Autodesk Fusion 360 part; units mm, degrees
sketch "Sketch1" plane through (0, 0, 0) normal (0, 1, 0) x (1, 0, 0)
  circle A0 centre (0, 0) radius 4.075
  line L0 (26.5, -2.5) -> (17.4, -2.5)
  line L1 (17.4, -2.5) -> (17.4, 2.5)
  line L2 (17.4, 2.5) -> (26.5, 2.5)
  line L3 (26.5, 2.5) -> (26.5, -2.5)
  line L4 (26.5, -2.5) -> (17.4, 2.5) construction
  line L5 (17.4, -2.5) -> (26.5, 2.5) construction
  circle A1 centre (13, 0) radius 2
  circle A2 centre (31, 0) radius 2
  line L6 (-10, 10) -> (41, 10)
  line L7 (41, 10) -> (41, -10)
  line L8 (41, -10) -> (-10, -10)
  line L9 (-10, -10) -> (-10, 10)
  line L10 (-10, 10) -> (-12, 10)
  line L11 (-12, 10) -> (-12, -10)
  line L12 (-12, -10) -> (-10, -10)
  line L13 (-10, -10) -> (-10, 10)
  line L14 (41, 10) -> (43, 10)
  line L15 (43, 10) -> (43, -10)
  line L16 (43, -10) -> (41, -10)
  line L17 (41, -10) -> (41, 10)
  point P0 (21.95, 0)
  dimension "d1" = 8.15
  dimension "d2" = 9.1
  dimension "d3" = 5
  dimension "d4" = 4
  dimension "d5" = 4
  dimension "d6" = 18
  dimension "d7" = 9.05
  dimension "d9" = 13
  dimension "d10" = 10
  dimension "d11" = 10
  dimension "d12" = 10
  dimension "d13" = 10
  dimension "d16" = 51
extrude "Extrude2" add sketch "Sketch1" along normal blind 2 contours L6 L7 L8 L9 L13 L17 makes body 1
extrude "Extrude1" add sketch "Sketch1" along normal blind 2 separate body contours L6 L7 L8 L9 L13 L17 makes body 2
extrude "Extrude3" add sketch "Sketch1" along normal blind 55 contours L9 L10 L11 L12 L13 | L7 L14 L15 L16 L17 bodies 1 2
sketch "Sketch2" plane through (-10, 0, 0) normal (1, 0, 0) x (0, 0, -1)
  line L0 (-10, 2) -> (10, 2)
  line L1 (10, 2) -> (10, 55)
  line L2 (10, 55) -> (-10, 55)
  line L3 (-10, 55) -> (-10, 2)
  line L4 (-10, 55) -> (10, 55)
  line L5 (10, 55) -> (10, 53)
  line L6 (10, 53) -> (-10, 53)
  line L7 (-10, 53) -> (-10, 55)
  dimension "d21" = 2
extrude "Extrude4" add sketch "Sketch2" along normal up to surface (51 mm away) contours L1 L2 L3 L4 L5 L6 L7 bodies 1
sketch "Sketch3" plane through (0, 0, 10) normal (0, 0, 1) x (1, 0, 0)
  line L0 (41, 53) -> (41, 2)
  line L1 (41, 2) -> (-10, 2)
  line L2 (-10, 2) -> (-10, 53)
  line L3 (-10, 53) -> (41, 53)
  line L4 (43, 55) -> (-12, 55)
  line L5 (-12, 55) -> (-12, 0)
  line L6 (-12, 0) -> (43, 0)
  line L7 (43, 0) -> (43, 55)
extrude "Extrude5" add sketch "Sketch3" along normal blind 2 contours L0 L1 L2 L3 | L4 L5 L6 L7 bodies 1
sketch "Sketch4" plane through (0, 0, -10) normal (0, 0, -1) x (-1, 0, 0)
  line L0 (12, 55) -> (-43, 55)
  line L1 (-43, 55) -> (-43, 0)
  line L2 (-43, 0) -> (12, 0)
  line L3 (12, 0) -> (12, 55)
  line L4 (-41, 53) -> (10, 53)
  line L5 (10, 53) -> (10, 2)
  line L6 (10, 2) -> (-41, 2)
  line L7 (-41, 2) -> (-41, 53)
extrude "Extrude6" add sketch "Sketch4" along normal blind 14 bodies 1
sketch "Sketch5" plane through (43, 0, 0) normal (1, 0, 0) x (0, 0, -1)
  line L0 (-12, 0) -> (24, 0)
  line L1 (24, 0) -> (24, 55)
  line L2 (24, 55) -> (-12, 55)
  line L3 (-12, 55) -> (-12, 0)
  line L4 (24, 55) -> (22, 55)
  line L5 (22, 55) -> (22, 0)
  line L6 (22, 0) -> (24, 0)
  line L7 (24, 0) -> (24, 55)
extrude "Extrude7" add sketch "Sketch5" along normal blind 5 contours L0 L1 L2 L4 L5 L6 L7 bodies 1
sketch "Sketch6" plane through (-12, 0, 0) normal (-1, 0, 0) x (0, 0, 1)
  line L0 (-24, 0) -> (12, 0)
  line L1 (12, 0) -> (12, 55)
  line L2 (12, 55) -> (-24, 55)
  line L3 (-24, 55) -> (-24, 0)
  line L4 (-24, 55) -> (-22, 55)
  line L5 (-22, 55) -> (-22, 0)
  line L6 (-22, 0) -> (-24, 0)
  line L7 (-24, 0) -> (-24, 55)
  point P0 (-22, 0)
extrude "Extrude8" add sketch "Sketch6" along normal blind 5 contours L0 L2 L3 L4 L5 L6 L7 bodies 1
sketch "Sketch7" plane through (0, 55, 0) normal (0, 1, 0) x (-1, 0, 0)
  line L0 (-48, -24) -> (17, -24)
  line L1 (17, -24) -> (17, -22)
  line L2 (17, -22) -> (12, -22)
  line L3 (12, -22) -> (12, 12)
  line L4 (12, 12) -> (-43, 12)
  line L5 (-43, 12) -> (-43, -22)
  line L6 (-43, -22) -> (-48, -22)
  line L7 (-48, -22) -> (-48, -24)
  line L8 (17, -22) -> (-48, -22)
  line L9 (-48, -22) -> (-48, -24)
  line L10 (-48, -24) -> (17, -24)
  line L11 (17, -24) -> (17, -22)
extrude "Extrude9" add sketch "Sketch7" along normal blind 5 contours L0 L1 L2 L6 L7 L8 L9 L10 L11 bodies 1
sketch "Sketch8" plane through (0, 0, 0) normal (0, -1, 0) x (1, 0, 0)
  circle A0 centre (0, 0) radius 4.075
  circle A1 centre (31, 0) radius 2
  line L0 (26.5, -2.5) -> (17.4, -2.5)
  line L1 (17.4, -2.5) -> (17.4, 2.5)
  line L2 (17.4, 2.5) -> (26.5, 2.5)
  line L3 (26.5, 2.5) -> (26.5, -2.5)
  circle A2 centre (13, 0) radius 2
  line L4 (-12, 12) -> (-12, -22)
  line L5 (-12, -22) -> (-17, -22)
  line L6 (-17, -22) -> (-17, -24)
  line L7 (-17, -24) -> (48, -24)
  line L8 (48, -24) -> (48, -22)
  line L9 (48, -22) -> (43, -22)
  line L10 (43, -22) -> (43, 12)
  line L11 (43, 12) -> (-12, 12)
  line L12 (-17, -24) -> (48, -24)
  line L13 (48, -24) -> (48, -22)
  line L14 (48, -22) -> (-17, -22)
  line L15 (-17, -22) -> (-17, -24)
extrude "Extrude10" add sketch "Sketch8" along normal blind 5 contours L5 L6 L7 L8 L9 L12 L13 L14 L15 bodies 1
chamfer "Chamfer1" distance 2 angle 45 4 edges at (-17, 27.5, -24) (15.5, 60, -24) (48, 27.5, -24) (15.5, -5, -24) on bodies 1
sketch "Sketch9" plane through (0, 0, 0) normal (0, 1, 0) x (-1, 0, 0)
sketch "Sketch10" plane through (0, 0, 12) normal (0, 0, 1) x (1, 0, 0)
  line L0 (43, 0) -> (43, 55)
  line L1 (43, 55) -> (-12, 55)
  line L2 (-12, 55) -> (-12, 0)
  line L3 (-12, 0) -> (43, 0)
  line L4 (19.95, 20.95) -> (19.95, 30.05)
  line L5 (19.95, 30.05) -> (24.95, 30.05)
  line L6 (24.95, 30.05) -> (24.95, 20.95)
  line L7 (24.95, 20.95) -> (19.95, 20.95)
  circle A0 centre (22.45, 16.45) radius 2
  circle A1 centre (22.45, 34.45) radius 2
  dimension "d37" = 9.1
  dimension "d38" = 5
  dimension "d39" = 4
  dimension "d40" = 4
  dimension "d41" = 18
extrude "Extrude11" cut sketch "Sketch10" against normal blind 2 contours L4 L5 L6 L7 | A0 | A1 bodies 1
extrude "Extrude12" add sketch "Sketch1" along normal blind 2 contours L0 L1 L2 L3 | A1 | A2 bodies 1
For this review, take the finished solid that the model builds, in its own axes (mm). A direction names the side the tool comes from. Coordinates: 2 decimals unless noted, no trailing zeros. Loops run counter-clockwise (first coordinate to the right, second up) from the corner with the lowest first, then second, coordinate; pieces in that order, holes last. Notation, with made-up numbers: (23.5, -38) -> (34.5, -38) arc R11 ccw to (34.5, -27) -> close; hole circle Ø5 at (35.25, 57). An arc over 180 degrees is marked (long way). Return JSON: item names as keys, results as strings. Group by question number.
(1) Tool access review of faces 1 (the flat face through (-10, 28, -7)), 2 (the flat face through (16, 0, -5)), 3 (the flat face through (43, 28, -5)), 4 (the flat face through (22, 20.95, 11)): name each direction out of +Z, -Z, +X, -X, +Y, -Y from which nothing blocks a thin tool from reaching the whole face with its end or side.
(2) Mouldability with a two-part tool opening along Z and no side actions: class faces 5 (the flat face through (15, 59, -23)), 6 (the flat face through (15, 28, 12)), 7 (the cylindrical face through (-3.234, 0.986, -2.48)), 8 (the flat face through (15, 2, -7)) as pulls with the +Z half, pulls with the -Z half, needs draft (parallel to the pull), parting line crosses it, or undercut.
(3) Consider section B-B, the plane x = 22.45. Count the separate pieces of the cut face and the enclosed holes in it, plus the area to 3 significant figures.
(4) For pin 1 Ø0.6 at (y, z) = (26, 10.5) entering from +X; pin 2 Ø4 at (x, z) = (25.5, -9.5) entering from -Y; pin 3 Ø3 at (x, z) = (0, -18.5) entering from +Y; pin 4 Ø10 at (x, y) = (22.5, 4) entering from -Z, all flat-tipped, find the tip position at first contact; note any pin that passes through.
(5) Consider section C-C, the plane z = 0. Give the boundary of the cut face in (x, y) (3 decimals), plus the area to 3 significant figures.
(6) To check wall thickness, follow L1, parallel to Y at x = 22.45, z = 10.5; L2, parallel to X at y = 36.5, z = -9.5; L3, parallel to Y at x = 7, z = -19. State the ranges of each line that lie inside material, in increasing order.
Results below:
{
 "1": {"face 1": "-Z", "face 2": "+Z, +X, -X, -Y", "face 3": "+Z, +X, +Y, -Y", "face 4": "+Z, -Z"},
 "2": {"face 5": "pulls with the -Z half", "face 6": "pulls with the +Z half", "face 7": "undercut", "face 8": "needs draft"},
 "3": {"separate pieces": "4", "enclosed holes": "0", "area": "228 mm2"},
 "4": {"pin 1": "stops at x = 43", "pin 2": "stops at y = 0", "pin 3": "stops at y = 55", "pin 4": "stops at z = -24"},
 "5": {"outline": "(-12, 0) -> (-4.075, 0) -> (-4.075, 2) -> (-10, 2) -> (-10, 53) -> (41, 53) -> (41, 2) -> (4.075, 2) -> (4.075, 0) -> (43, 0) -> (43, 55) -> (-12, 55) -> close", "area": "408 mm2"},
 "6": {"L1": "y = 0 to 14.45, 18.45 to 20.95, 30.05 to 32.45, 36.45 to 55", "L2": "x = -12 to -10, 41 to 43", "L3": "y = 0 to 2, 53 to 55"}
}
